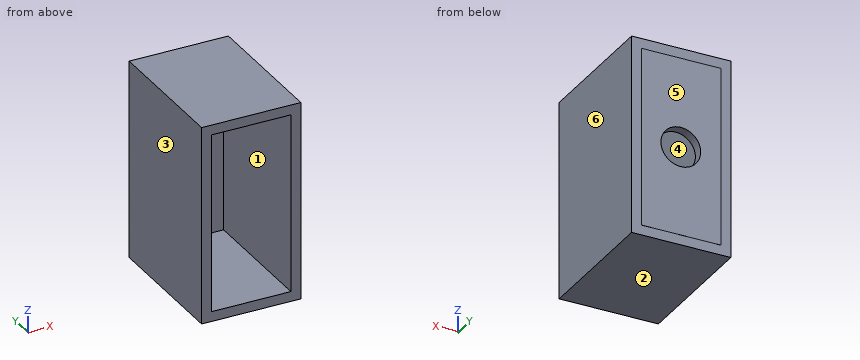
```python
from build123d import *

# Parameters (mm, degrees)
SKETCH1_W                = 50.8
SKETCH1_H                = 101.6
SKETCH1_W_2              = 40.64
SKETCH1_H_2              = 91.44
BOSS_EXTRUDE1_DEPTH      = 70.61
BOSS_EXTRUDE2_DEPTH      = 0.0254
BOSS_EXTRUDE2_DEPTH_BACK = 5.08
SKETCH2_W                = 40.64
SKETCH2_H                = 91.44
SKETCH3_R                = 10.171709971
CUT_EXTRUDE1_DEPTH       = 106.159035776


with BuildPart() as part:
    # Sketch1 → Boss-Extrude1 (new body)
    with BuildSketch(Plane(origin=(0, 0, 0), x_dir=(1, 0, 0), z_dir=(0, 1, 0))):
        with Locations((-0.241139241, -22.763544304)):
            Rectangle(SKETCH1_W, SKETCH1_H)
        with Locations((-0.241139241, -22.763544304)):
            Rectangle(SKETCH1_W_2, SKETCH1_H_2, mode=Mode.SUBTRACT)
    extrude(amount=BOSS_EXTRUDE1_DEPTH)

    # Sketch2 → Boss-Extrude2 (add, two sides: drawn at the far end of the back side and taken through both)
    with BuildSketch(Plane(origin=(0, 70.61, 0), x_dir=(1, 0, 0), z_dir=(0, 1, 0)).offset(-BOSS_EXTRUDE2_DEPTH_BACK)):
        with Locations((-0.241139241, -22.763544304)):
            Rectangle(SKETCH2_W, SKETCH2_H)
    extrude(amount=BOSS_EXTRUDE2_DEPTH + BOSS_EXTRUDE2_DEPTH_BACK)

    # Sketch3 → Cut-Extrude1 (cut, through all)
    with BuildSketch(Plane(origin=(0, 70.6354, 0), x_dir=(1, 0, 0), z_dir=(0, 1, 0))):
        with Locations(Location((0, -22.565616606, 0), (0, 0, 270))):
            Circle(SKETCH3_R)
    extrude(amount=-CUT_EXTRUDE1_DEPTH, mode=Mode.SUBTRACT)


solid = part.part
```
Verification items for the finished model (mm, model axes). Face numbers are marked on the shaded views. A direction names the side the tool comes from. Give positions to 0.01 mm unless a question says otherwise; leave off trailing zeros. Order: outer loops, then holes, each group sorted by start corner. A loop starts at its lowest first (then second) coordinate and runs counter-clockwise, first axis right, second up. Notation, with made-up numbers: M -14,2.5 L 23,2.5 A23 ccw 23,18.5 Z; hole C -28,-34 d3. An arc over 180 degrees is marked long. Answer in a Markdown table with one row per item. Add a question column.
Item 1: Mould release check, pull along X, two halves, no side actions. Record for the marked faces 3, 4, 5 and 6: released by +X, released by -X, zero draft, split by the parting line, or undercut.
Item 2: Scan lines: probe 1 along Z at (x, y) = (-1, 49.5); probe 2 along X at (y, z) = (32, 9); probe 3 along Y at (x, z) = (19, -10.5). Record each from-to range of solid material in increasing order. Write a range as from..to.
Item 3: Section check B-B, the plane y = 51. Enter the section's corners in (x, z).
Item 4: Tool access check on the marked faces 1 and 2. Record the directions out of +Z, -Z, +X, -X, +Y, -Y that give a thin tool (end or side, any length) a straight path to the whole face; none if there is none.
Item 5: Gauge pin test, flat end, axial feed: pin 1 (12 mm diameter, centred on x = 0, z = 22.57, fed in from +Y) (3 decimals). Record the tip position at first contact, or that the pin passes through.
Filled sheet:
| question | item | result |
|---|---|---|
| 1 | face 3 | released by -X |
| 1 | face 4 | undercut |
| 1 | face 5 | zero draft |
| 1 | face 6 | released by +X |
| 2 | probe 1 | z = -28.04..-22.96, 68.48..73.56 |
| 2 | probe 2 | x = -25.64..-20.56, 20.08..25.16 |
| 2 | probe 3 | y = 65.53..70.64 |
| 3 | outline | M -25.64,-28.04 L 25.16,-28.04 L 25.16,73.56 L -25.64,73.56 Z; hole M -20.56,-22.96 L 20.08,-22.96 L 20.08,68.48 L -20.56,68.48 Z |
| 4 | face 1 | -Y |
| 4 | face 2 | -Z, +X, -X, +Y, -Y |
| 5 | pin 1 | passes through |
